For this review, use the dimensioned drawing (mm, ordinates from the lowest corner) and the shaded views. A direction names the side the tool comes from. Coordinates: 2 decimals unless noted, no trailing zeros. Order: outer loops, then holes, each group sorted by start corner. A loop starts at its lowest first (then second) coordinate and runs counter-clockwise, first axis right, second up. Notation, with made-up numbers: M 21.5,-19 L 75.5,-19 A4 cw 75.5,-13 Z; hole C 88,-4.75 d5. An arc over 180 degrees is marked long. Answer as CSV lines item,"result". Start each with the question number.
Q1. Machinability: for the marked faces 5 and 6, which of the approach directions +Z, -Z, +X, -X, +Y, -Y give a long, thin tool a straight path to every point of the face, cutting with its end or side? Answer none if there is none.
Q2. Wall thickness on L1, parallel to Z at x = 42, y = 44; L2, parallel to X at y = 42, z = 26.5; L3, parallel to X at y = 45.25, z = 24: over which ranges is each line inside the solid? List them lowest first. Write a range as [from, to].
Q3. Consider section D-D on y = 25. Write out the cut boundary in (x, z).
Q4. Consider section A-A on y = 42. Write out the cut boundary in (x, z).
Q5. For P1, Ø1.5, axis at x = 42, z = 24, coming from the -Y side; P2, Ø3.5, axis at x = 30, y = 42, coming from the -Z side; P3, Ø4, axis at x = 41, z = 13, coming from the +Y side, all flat-tipped, find the tip position at first contact; note any pin that passes through.
Q6. Consider section C-C on x = 22. Write out the cut boundary in (y, z), and give its area (3 significant figures).
Q7. The part is to be moulded in two halves that separate along Y. For the marked faces 1, 2, 3 and 4, say which applies: +Y half, -Y half, draft (parallel to the pull), parting line (faces both ways), or undercut.
Q8. Consider section B-B on z = 15. Write out the cut boundary in (x, y), and give its area (3 significant figures).
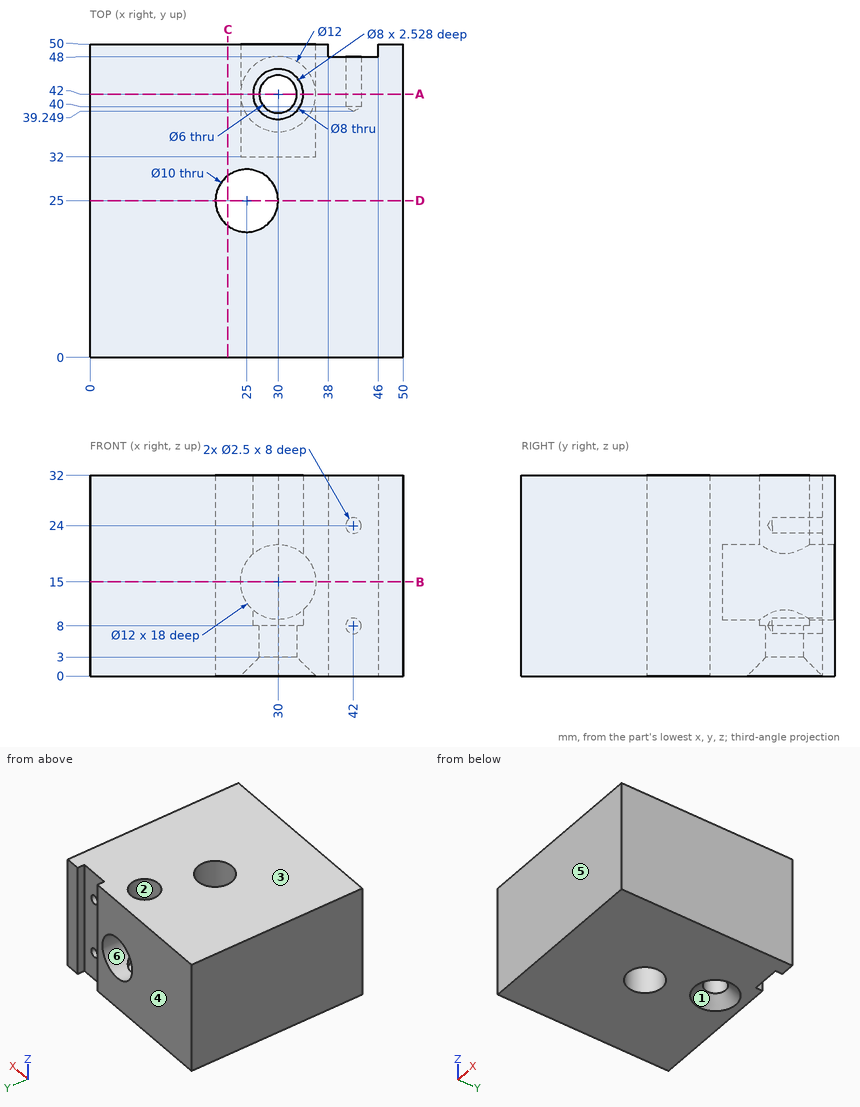
Evaluation:
1,face 5,"+Z, -Z, +X, -X, -Y"
1,face 6,"+Y"
2,L1,"z = [0, 6.75], [9.25, 22.75], [25.25, 32]"
2,L2,"x = [0, 26], [34, 50]"
2,L3,"x = [0, 27.67], [32.33, 40.75], [43.25, 50]"
3,outline,"M 0,0 L 20,0 L 20,32 L 0,32 Z; M 30,0 L 50,0 L 50,32 L 30,32 Z"
4,outline,"M 0,0 L 24,0 L 27,3 L 27,8 L 26,8 L 26,10.53 A6 cw 26,19.47 L 26,32 L 0,32 Z; M 33,3 L 36,0 L 50,0 L 50,32 L 34,32 L 34,19.47 A6 cw 34,10.53 L 34,8 L 33,8 Z; hole C 42,8 d2.5; hole C 42,24 d2.5"
5,P1,"stops at y = 0"
5,P2,"passes through"
5,P3,"stops at y = 48"
6,outline,"M 0,0 L 21,0 L 21,32 L 0,32 Z; M 29,0 L 50,0 L 50,32 L 29,32 Z"
6,area,"1,340 mm²"
7,face 1,"undercut"
7,face 2,"undercut"
7,face 3,"draft"
7,face 4,"+Y half"
8,outline,"M 0,0 L 50,0 L 50,50 L 46,50 L 46,48 L 38,48 L 38,50 L 36,50 L 36,32 L 24,32 L 24,50 L 0,50 Z; hole C 25,25 d10"
8,area,"2,190 mm²"
